Here's how the part is built. I have some questions about the finished solid (model axes, mm). Face numbers are marked on the shaded views. A direction names the side the tool comes from. Give positions to 0.01 mm unless a question says otherwise; leave off trailing zeros. Write each loop counter-clockwise with the first axis right and the second up, starting at its lowest first coordinate (ties: lowest second). Pieces come first, ordered by that corner, then holes. Notation, with made-up numbers: (68, 57) - (84, 57) arc R9 ccw to (84, 69) - close; hole circle Ø1 at (10.5, 32.5). An arc over 180 degrees is marked (long way). Use a Markdown table: item, result.
```python
from build123d import *

# Parameters (mm, degrees)
SKETCH1_W               = 72
SKETCH1_H               = 42
SKETCH1_W_2             = 68
SKETCH1_H_2             = 38
BOSS_EXTRUDE1_DEPTH     = 2
BOSS_EXTRUDE2_START     = 2
SKETCH1_3_W             = 72
SKETCH1_3_H             = 42
SKETCH1_3_W_2           = 68
SKETCH1_3_H_2           = 38
BOSS_EXTRUDE2_DEPTH     = 14
CHAMFER1_SIZE           = 2
SKETCH2_R               = 1.25
BOSS_EXTRUDE3_DEPTH     = 2
MIRROR2_COPY_1_SKETCH_R = 1.25
MIRROR2_COPY_1_DEPTH    = 2
CUT_EXTRUDE1_DEPTH      = 1.6
MIRROR4_COPY_1_DEPTH    = 1.6
CUT_EXTRUDE2_DEPTH      = 44.965895874
CUT_EXTRUDE2_DEPTH_BACK = 44.965895874
SKETCH4_R               = 1.25
SKETCH5_W               = 7.5
SKETCH5_H               = 2
CUT_EXTRUDE3_DEPTH      = 1
CUT_EXTRUDE3_DRAFT      = -38
MIRROR5_COPY_1_SKETCH_W = 7.5
MIRROR5_COPY_1_SKETCH_H = 2
MIRROR5_COPY_1_DEPTH    = 1
MIRROR5_COPY_1_DRAFT    = -38
MIRROR8_COPY_1_SKETCH_W = 7.5
MIRROR8_COPY_1_SKETCH_H = 2
MIRROR8_COPY_1_DEPTH    = 1
MIRROR8_COPY_1_DRAFT    = -38
MIRROR8_COPY_2_SKETCH_W = 7.5
MIRROR8_COPY_2_SKETCH_H = 2
MIRROR8_COPY_2_DEPTH    = 1
MIRROR8_COPY_2_DRAFT    = -38
SKETCH6_W               = 5
SKETCH6_H               = 2
CUT_EXTRUDE4_DEPTH      = 1
CUT_EXTRUDE4_DRAFT      = -38
MIRROR6_COPY_1_SKETCH_W = 5
MIRROR6_COPY_1_SKETCH_H = 2
MIRROR6_COPY_1_DEPTH    = 1
MIRROR6_COPY_1_DRAFT    = -38
MIRROR7_COPY_1_SKETCH_W = 5
MIRROR7_COPY_1_SKETCH_H = 2
MIRROR7_COPY_1_DEPTH    = 1
MIRROR7_COPY_1_DRAFT    = -38
MIRROR7_COPY_2_SKETCH_W = 5
MIRROR7_COPY_2_SKETCH_H = 2
MIRROR7_COPY_2_DEPTH    = 1
MIRROR7_COPY_2_DRAFT    = -38
SKETCH7_W               = 11
SKETCH7_H               = 7.5
CUT_EXTRUDE5_DEPTH      = 77.68767828


with BuildPart() as part:
    # Sketch1 → Boss-Extrude1 (new body)
    # profile 1 of 2: a face of its own
    with BuildSketch(Plane(origin=(0, 0, 0), x_dir=(1, 0, 0), z_dir=(0, 1, 0))):
        Rectangle(SKETCH1_W, SKETCH1_H)
        Rectangle(SKETCH1_W_2, SKETCH1_H_2, mode=Mode.SUBTRACT)
    # profile 2 of 2: a face of its own
    with BuildSketch(Plane(origin=(0, 0, 0), x_dir=(1, 0, 0), z_dir=(0, 1, 0))):
        Rectangle(SKETCH1_W_2, SKETCH1_H_2)
    extrude(amount=BOSS_EXTRUDE1_DEPTH)

    # Sketch1<3> → Boss-Extrude2 (add)
    with BuildSketch(Plane(origin=(0, 0, 0), x_dir=(1, 0, 0), z_dir=(0, 1, 0)).offset(BOSS_EXTRUDE2_START)):
        Rectangle(SKETCH1_3_W, SKETCH1_3_H)
        Rectangle(SKETCH1_3_W_2, SKETCH1_3_H_2, mode=Mode.SUBTRACT)
    extrude(amount=BOSS_EXTRUDE2_DEPTH)

    # Chamfer1
    chamfer1_edges = [part.edges().sort_by_distance(p)[0] for p in [
        (0, 0, -21),
        (36, 0, 0),
        (0, 0, 21),
        (-36, 0, 0),
        (-36, 8, -21),
        (36, 8, -21),
        (36, 8, 21),
        (-36, 8, 21),
    ]]
    chamfer(chamfer1_edges, length=CHAMFER1_SIZE)

    # Sketch2 → Boss-Extrude3 (add)
    with BuildSketch(Plane(origin=(0, 2, 0), x_dir=(1, 0, 0), z_dir=(0, 1, 0))):
        with BuildLine():
            Line((-34, 12), (-30, 12))
            ThreePointArc((-30, 12), (-27.878679656, 12.878679656), (-27, 15))
            Line((-27, 15), (-27, 19))
            Line((-27, 19), (-34, 19))
            Line((-34, 19), (-34, 12))
        make_face()
        with Locations(Location((-30.5, 15.5, 0), (0, 0, 270))):
            Circle(SKETCH2_R, mode=Mode.SUBTRACT)
    boss_extrude3 = extrude(amount=BOSS_EXTRUDE3_DEPTH)

    # Mirror1: Boss-Extrude3 across plane
    add(boss_extrude3.mirror(Plane.XY))

    # Mirror2: Boss-Extrude3 across plane
    add(boss_extrude3.mirror(Plane(origin=(0, 0, 0), x_dir=(0, 0, 1), z_dir=(1, 0, 0))))

    # Mirror2 copy 1 sketch → Mirror2 copy 1 (add)
    with BuildSketch(Plane(origin=(0, 2, 0), x_dir=(-1, 0, 0), z_dir=(0, 1, 0))):
        with BuildLine():
            Line((-34, 12), (-30, 12))
            ThreePointArc((-30, 12), (-27.878679656, 12.878679656), (-27, 15))
            Line((-27, 15), (-27, 19))
            Line((-27, 19), (-34, 19))
            Line((-34, 19), (-34, 12))
        make_face()
        with Locations(Location((-30.5, 15.5, 0), (0, 0, 270))):
            Circle(MIRROR2_COPY_1_SKETCH_R, mode=Mode.SUBTRACT)
    extrude(amount=MIRROR2_COPY_1_DEPTH)

    # Sketch3 → Cut-Extrude1 (cut)
    with BuildSketch(Plane.XZ):
        Polygon((-31.799038106, 17.75), (-29.200961894, 17.75), (-27.901923789, 15.5), (-29.200961894, 13.25), (-31.799038106, 13.25), (-33.098076211, 15.5), align=None)
    cut_extrude1 = extrude(amount=-CUT_EXTRUDE1_DEPTH, mode=Mode.SUBTRACT)

    # Mirror3: Cut-Extrude1 across plane
    add(cut_extrude1.mirror(Plane.XY), mode=Mode.SUBTRACT)

    # Mirror4: Cut-Extrude1 across plane
    add(cut_extrude1.mirror(Plane(origin=(0, 0, 0), x_dir=(0, 0, 1), z_dir=(1, 0, 0))), mode=Mode.SUBTRACT)

    # Mirror4 copy 1 sketch → Mirror4 copy 1 (cut)
    with BuildSketch(Plane(origin=(0, 0, 0), x_dir=(-1, 0, 0), z_dir=(0, -1, 0))):
        Polygon((-31.799038106, 17.75), (-29.200961894, 17.75), (-27.901923789, 15.5), (-29.200961894, 13.25), (-31.799038106, 13.25), (-33.098076211, 15.5), align=None)
    extrude(amount=-MIRROR4_COPY_1_DEPTH, mode=Mode.SUBTRACT)

    # Sketch4 → Cut-Extrude2 (cut, two sides: drawn at the far end of the back side and taken through both)
    with BuildSketch(Plane(origin=(0, 2, 0), x_dir=(1, 0, 0), z_dir=(0, 1, 0)).offset(-CUT_EXTRUDE2_DEPTH_BACK)):
        with Locations(Location((30.5, -15.5, 0), (0, 0, 90))):
            Circle(SKETCH4_R)
        with Locations(Location((30.5, 15.5, 0), (0, 0, 270))):
            Circle(SKETCH4_R)
        with Locations(Location((-30.5, 15.5, 0), (0, 0, 270))):
            Circle(SKETCH4_R)
        with Locations(Location((-30.5, -15.5, 0), (0, 0, 90))):
            Circle(SKETCH4_R)
    extrude(amount=CUT_EXTRUDE2_DEPTH + CUT_EXTRUDE2_DEPTH_BACK, mode=Mode.SUBTRACT)


with BuildPart() as cut_extrude3_tool:
    # Sketch5 → Cut-Extrude3 (with draft: the straight prism first)
    with BuildSketch(Plane(origin=(0, 0, 19), x_dir=(-1, 0, 0), z_dir=(0, 0, -1))):
        with Locations((-20.25, 14)):
            Rectangle(SKETCH5_W, SKETCH5_H)
    extrude(amount=-CUT_EXTRUDE3_DEPTH)
    # Cut-Extrude3: the draft: its side faces are tilted about the plane it starts from
    cut_extrude3_sides = [cut_extrude3_tool.faces().sort_by_distance(p)[0] for p in [
        (24, 14, 19.5),
        (20.25, 13, 19.5),
        (16.5, 14, 19.5),
        (20.25, 15, 19.5),
    ]]
    draft(cut_extrude3_sides, Plane(origin=(0, 0, 19), x_dir=(-1, 0, 0), z_dir=(0, 0, -1)), CUT_EXTRUDE3_DRAFT)


with BuildPart() as part_1:
    add(part.part)

    # Cut-Extrude3: cut by cut_extrude3_tool
    add(cut_extrude3_tool.part, mode=Mode.SUBTRACT)


with BuildPart() as mirror5_copy_1_tool:
    # Mirror5 copy 1 sketch → Mirror5 copy 1 (with draft: the straight prism first)
    with BuildSketch(Plane(origin=(0, 0, -19), x_dir=(-1, 0, 0), z_dir=(0, 0, 1))):
        with Locations((-20.25, -14)):
            Rectangle(MIRROR5_COPY_1_SKETCH_W, MIRROR5_COPY_1_SKETCH_H)
    extrude(amount=-MIRROR5_COPY_1_DEPTH)
    # Mirror5 copy 1: the draft: its side faces are tilted about the plane it starts from
    mirror5_copy_1_sides = [mirror5_copy_1_tool.faces().sort_by_distance(p)[0] for p in [
        (24, 14, -19.5),
        (20.25, 13, -19.5),
        (16.5, 14, -19.5),
        (20.25, 15, -19.5),
    ]]
    draft(mirror5_copy_1_sides, Plane(origin=(0, 0, -19), x_dir=(-1, 0, 0), z_dir=(0, 0, 1)), MIRROR5_COPY_1_DRAFT)


with BuildPart() as part_2:
    add(part_1.part)

    # Mirror5 copy 1: cut by mirror5_copy_1_tool
    add(mirror5_copy_1_tool.part, mode=Mode.SUBTRACT)


with BuildPart() as mirror8_copy_1_tool:
    # Mirror8 copy 1 sketch → Mirror8 copy 1 (with draft: the straight prism first)
    with BuildSketch(Plane(origin=(0, 0, 19), x_dir=(1, 0, 0), z_dir=(0, 0, -1))):
        with Locations((-20.25, -14)):
            Rectangle(MIRROR8_COPY_1_SKETCH_W, MIRROR8_COPY_1_SKETCH_H)
    extrude(amount=-MIRROR8_COPY_1_DEPTH)
    # Mirror8 copy 1: the draft: its side faces are tilted about the plane it starts from
    mirror8_copy_1_sides = [mirror8_copy_1_tool.faces().sort_by_distance(p)[0] for p in [
        (-24, 14, 19.5),
        (-20.25, 13, 19.5),
        (-16.5, 14, 19.5),
        (-20.25, 15, 19.5),
    ]]
    draft(mirror8_copy_1_sides, Plane(origin=(0, 0, 19), x_dir=(1, 0, 0), z_dir=(0, 0, -1)), MIRROR8_COPY_1_DRAFT)


with BuildPart() as part_3:
    add(part_2.part)

    # Mirror8 copy 1: cut by mirror8_copy_1_tool
    add(mirror8_copy_1_tool.part, mode=Mode.SUBTRACT)


with BuildPart() as mirror8_copy_2_tool:
    # Mirror8 copy 2 sketch → Mirror8 copy 2 (with draft: the straight prism first)
    with BuildSketch(Plane.XY.offset(-19)):
        with Locations((-20.25, 14)):
            Rectangle(MIRROR8_COPY_2_SKETCH_W, MIRROR8_COPY_2_SKETCH_H)
    extrude(amount=-MIRROR8_COPY_2_DEPTH)
    # Mirror8 copy 2: the draft: its side faces are tilted about the plane it starts from
    mirror8_copy_2_sides = [mirror8_copy_2_tool.faces().sort_by_distance(p)[0] for p in [
        (-24, 14, -19.5),
        (-20.25, 13, -19.5),
        (-16.5, 14, -19.5),
        (-20.25, 15, -19.5),
    ]]
    draft(mirror8_copy_2_sides, Plane.XY.offset(-19), MIRROR8_COPY_2_DRAFT)


with BuildPart() as part_4:
    add(part_3.part)

    # Mirror8 copy 2: cut by mirror8_copy_2_tool
    add(mirror8_copy_2_tool.part, mode=Mode.SUBTRACT)


with BuildPart() as cut_extrude4_tool:
    # Sketch6 → Cut-Extrude4 (with draft: the straight prism first)
    with BuildSketch(Plane(origin=(-34, 0, 0), x_dir=(0, 0, -1), z_dir=(1, 0, 0))):
        with Locations((-12.5, 14)):
            Rectangle(SKETCH6_W, SKETCH6_H)
    extrude(amount=-CUT_EXTRUDE4_DEPTH)
    # Cut-Extrude4: the draft: its side faces are tilted about the plane it starts from
    cut_extrude4_sides = [cut_extrude4_tool.faces().sort_by_distance(p)[0] for p in [
        (-34.5, 14, 15),
        (-34.5, 13, 12.5),
        (-34.5, 14, 10),
        (-34.5, 15, 12.5),
    ]]
    draft(cut_extrude4_sides, Plane(origin=(-34, 0, 0), x_dir=(0, 0, -1), z_dir=(1, 0, 0)), CUT_EXTRUDE4_DRAFT)


with BuildPart() as part_5:
    add(part_4.part)

    # Cut-Extrude4: cut by cut_extrude4_tool
    add(cut_extrude4_tool.part, mode=Mode.SUBTRACT)


with BuildPart() as mirror6_copy_1_tool:
    # Mirror6 copy 1 sketch → Mirror6 copy 1 (with draft: the straight prism first)
    with BuildSketch(Plane(origin=(34, 0, 0), x_dir=(0, 0, -1), z_dir=(-1, 0, 0))):
        with Locations((-12.5, -14)):
            Rectangle(MIRROR6_COPY_1_SKETCH_W, MIRROR6_COPY_1_SKETCH_H)
    extrude(amount=-MIRROR6_COPY_1_DEPTH)
    # Mirror6 copy 1: the draft: its side faces are tilted about the plane it starts from
    mirror6_copy_1_sides = [mirror6_copy_1_tool.faces().sort_by_distance(p)[0] for p in [
        (34.5, 14, 15),
        (34.5, 13, 12.5),
        (34.5, 14, 10),
        (34.5, 15, 12.5),
    ]]
    draft(mirror6_copy_1_sides, Plane(origin=(34, 0, 0), x_dir=(0, 0, -1), z_dir=(-1, 0, 0)), MIRROR6_COPY_1_DRAFT)


with BuildPart() as part_6:
    add(part_5.part)

    # Mirror6 copy 1: cut by mirror6_copy_1_tool
    add(mirror6_copy_1_tool.part, mode=Mode.SUBTRACT)


with BuildPart() as mirror7_copy_1_tool:
    # Mirror7 copy 1 sketch → Mirror7 copy 1 (with draft: the straight prism first)
    with BuildSketch(Plane(origin=(-34, 0, 0), x_dir=(0, 0, 1), z_dir=(1, 0, 0))):
        with Locations((-12.5, -14)):
            Rectangle(MIRROR7_COPY_1_SKETCH_W, MIRROR7_COPY_1_SKETCH_H)
    extrude(amount=-MIRROR7_COPY_1_DEPTH)
    # Mirror7 copy 1: the draft: its side faces are tilted about the plane it starts from
    mirror7_copy_1_sides = [mirror7_copy_1_tool.faces().sort_by_distance(p)[0] for p in [
        (-34.5, 14, -15),
        (-34.5, 13, -12.5),
        (-34.5, 14, -10),
        (-34.5, 15, -12.5),
    ]]
    draft(mirror7_copy_1_sides, Plane(origin=(-34, 0, 0), x_dir=(0, 0, 1), z_dir=(1, 0, 0)), MIRROR7_COPY_1_DRAFT)


with BuildPart() as part_7:
    add(part_6.part)

    # Mirror7 copy 1: cut by mirror7_copy_1_tool
    add(mirror7_copy_1_tool.part, mode=Mode.SUBTRACT)


with BuildPart() as mirror7_copy_2_tool:
    # Mirror7 copy 2 sketch → Mirror7 copy 2 (with draft: the straight prism first)
    with BuildSketch(Plane.ZY.offset(-34)):
        with Locations((-12.5, 14)):
            Rectangle(MIRROR7_COPY_2_SKETCH_W, MIRROR7_COPY_2_SKETCH_H)
    extrude(amount=-MIRROR7_COPY_2_DEPTH)
    # Mirror7 copy 2: the draft: its side faces are tilted about the plane it starts from
    mirror7_copy_2_sides = [mirror7_copy_2_tool.faces().sort_by_distance(p)[0] for p in [
        (34.5, 14, -15),
        (34.5, 13, -12.5),
        (34.5, 14, -10),
        (34.5, 15, -12.5),
    ]]
    draft(mirror7_copy_2_sides, Plane.ZY.offset(-34), MIRROR7_COPY_2_DRAFT)


with BuildPart() as part_8:
    add(part_7.part)

    # Mirror7 copy 2: cut by mirror7_copy_2_tool
    add(mirror7_copy_2_tool.part, mode=Mode.SUBTRACT)

    # Sketch7 → Cut-Extrude5 (cut, through all)
    with BuildSketch(Plane(origin=(36, 0, 0), x_dir=(0, 0, -1), z_dir=(1, 0, 0))):
        with Locations((0, 8.5)):
            Rectangle(SKETCH7_W, SKETCH7_H)
    extrude(amount=-CUT_EXTRUDE5_DEPTH, mode=Mode.SUBTRACT)


solid = part_8.part
```
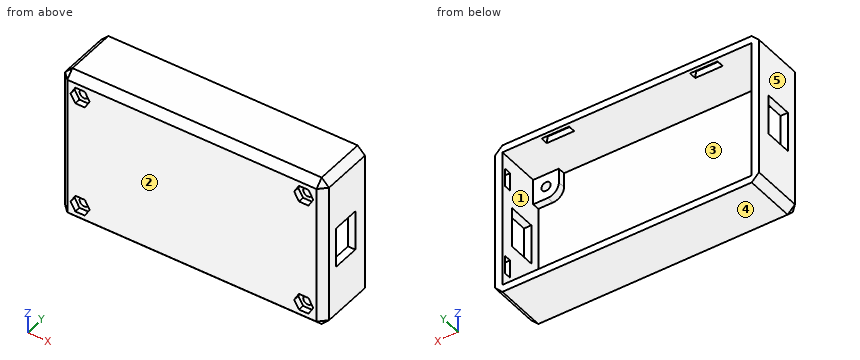
Item 1: For the marked faces 1 and 2, which set-ups out of +Z, -Z, +X, -X, +Y, -Y let a thin tool reach every point of the face, with its end or its side?
Values:
| item | result |
|---|---|
| face 1 | +Y |
| face 2 | +Z, -Z, +X, -X, -Y |
Item 2: I need wall thicknesses on line 1 along X through (y, z) = (2.4, 15.5); line 2 along X through (y, z) = (5, -16); line 3 along Z through (x, y) = (30.5, 2.75). Which ranges of each line are inside material? Lowest first, please. Write a range as [from, to].
Values:
| item | result |
|---|---|
| line 1 | x = [-36, -31.75], [-29.25, -27], [27, 29.25], [31.75, 36] |
| line 2 | x = [-36, -34], [34, 36] |
| line 3 | z = [-21, -16.75], [-14.25, -12], [12, 14.25], [16.75, 21] |
Item 3: If we section it at A-A, the plane y = 8.75: Write out the boundary of the cut face in (x, z).
Values:
| item | result |
|---|---|
| outline | (-36, -19) - (-34, -21) - (34, -21) - (36, -19) - (36, -5.5) - (34, -5.5) - (34, -19) - (-34, -19) - (-34, -5.5) - (-36, -5.5) - close; (-36, 5.5) - (-34, 5.5) - (-34, 19) - (34, 19) - (34, 5.5) - (36, 5.5) - (36, 19) - (34, 21) - (-34, 21) - (-36, 19) - close |
Item 4: Will these pins go through, and if not, where does the flat tip stop? pin 1 Ø5 at (y, z) = (9.5, -4.5) entering from +X; pin 2 Ø0.6 at (x, y) = (35, 9) entering from -Z; pin 3 Ø3 at (x, z) = (-30.5, 15.5) entering from +Y; pin 4 Ø1.8 at (x, y) = (-30, 1) entering from +Z.
Values:
| item | result |
|---|---|
| pin 1 | stops at x = 36 |
| pin 2 | stops at z = -20.3 |
| pin 3 | stops at y = 4 |
| pin 4 | stops at z = 20.9 |
Item 5: If we section it at C-C, the plane x = -8: Write out the boundary of the cut face in (y, z), plus the area to 3 significant figures.
Values:
| item | result |
|---|---|
| outline | (0, -19) - (2, -21) - (16, -21) - (16, -19) - (2, -19) - (2, 19) - (16, 19) - (16, 21) - (2, 21) - (0, 19) - close |
| area | 136 mm2 |
Item 6: Thinking about a two-plate mould opening in X: for the marked faces 3, 4 and 5, which applies, +X half, -X half, draft (parallel to the pull), parting line (faces both ways), or undercut?
Values:
| item | result |
|---|---|
| face 3 | undercut |
| face 4 | draft |
| face 5 | -X half |
Item 7: If we section it at B-B, the plane z = -3.5: Write out the boundary of the cut face in (x, y).
Values:
| item | result |
|---|---|
| outline | (-36, 2) - (-34, 0) - (34, 0) - (36, 2) - (36, 4.75) - (34, 4.75) - (34, 2) - (-34, 2) - (-34, 4.75) - (-36, 4.75) - close; (-36, 12.25) - (-34, 12.25) - (-34, 16) - (-36, 16) - close; (34, 12.25) - (36, 12.25) - (36, 16) - (34, 16) - close |
